```python
from build123d import *

# Parameters (mm, degrees)
SKETCH2_W           = 24
SKETCH2_H           = 75
BOSS_EXTRUDE1_DEPTH = 8
FILLET1_R           = 12
SKETCH3_W           = 24.000000014
SKETCH3_H           = 30
BOSS_EXTRUDE2_DEPTH = 50
SKETCH4_W           = 42
SKETCH4_H           = 27.227537437
CUT_EXTRUDE1_DEPTH  = 24
FILLET2_R           = 7
CUT_EXTRUDE3_DEPTH  = 14
SKETCH6_R           = 3
BOSS_EXTRUDE3_DEPTH = 5
FILLET3_R           = 3
SKETCH7_R           = 2
CUT_EXTRUDE4_DEPTH  = 102.473144681
SKETCH8_R           = 3
CUT_EXTRUDE5_DEPTH  = 4
SKETCH9_R           = 2
CUT_EXTRUDE6_DEPTH  = 10
FILLET4_R           = 7.5


# Some blends are built 0.0001 mm under size
with BuildPart() as part:
    # Sketch2 → Boss-Extrude1 (new body)
    with BuildSketch(Plane(origin=(0, -0.00023232, -27.997849314), x_dir=(1.0, -2.2299085471311813e-10, 0), z_dir=(-1.0101845712424022e-15, -8.29778911543011e-06, -0.9999999999655734))):
        with Locations((57.195219243, 10.372982491)):
            Rectangle(SKETCH2_W, SKETCH2_H)
    extrude(amount=BOSS_EXTRUDE1_DEPTH)

    # Fillet1
    # the kernel refuses this fillet: 12 mm, written as the material it takes off along each edge
    with BuildSketch(Plane(origin=(45.195219249, 27.127034112, 2.001925591), x_dir=(1.0, -2.229911070638136e-10, 0), z_dir=(-1.0101845712424022e-15, -8.29778911543011e-06, -0.9999999999655734))) as fillet1_piece_1:
        with BuildLine():
            CenterArc((FILLET1_R, FILLET1_R), FILLET1_R, 180, 90)
            Line((0, FILLET1_R), (0, 0))
            Line((0, 0), (FILLET1_R, 0))
        make_face()
    extrude(amount=68, mode=Mode.SUBTRACT)
    with BuildSketch(Plane(origin=(69.195219249, 27.127034106, 2.001925591), x_dir=(-1.0, 2.229905149399539e-10, 0), z_dir=(-1.0101845712424022e-15, -8.29778911543011e-06, -0.9999999999655734))) as fillet1_piece_2:
        with BuildLine():
            CenterArc((FILLET1_R, -FILLET1_R), FILLET1_R, 90, 90)
            Line((0, -FILLET1_R), (0, 0))
            Line((0, 0), (FILLET1_R, 0))
        make_face()
    extrude(amount=68, mode=Mode.SUBTRACT)

    # Sketch3 → Boss-Extrude2 (add)
    with BuildSketch(Plane(origin=(0, -0.00023232, -27.997849314), x_dir=(1, 0, 0), z_dir=(0, 8.297789115425485e-06, 0.9999999999655734))):
        with Locations((57.19521924, -32.872982501)):
            Rectangle(SKETCH3_W, SKETCH3_H)
    extrude(amount=BOSS_EXTRUDE2_DEPTH)

    # Sketch4 → Cut-Extrude1 (cut)
    with BuildSketch(Plane(origin=(69.195219243, -1.5e-08, 0), x_dir=(0, 0, -1), z_dir=(1.0, -2.2299088501705893e-10, 0))):
        with Locations((6.99770101, -40.486956155)):
            Rectangle(SKETCH4_W, SKETCH4_H)
    extrude(amount=-CUT_EXTRUDE1_DEPTH, mode=Mode.SUBTRACT)

    # Fillet2
    fillet2_edges = [part.edges().sort_by_distance(p)[0] for p in [
        (57.19521924, -17.87321482, -27.997701008),
        (57.19521924, -17.872799931, 22.002298991),
    ]]
    fillet(fillet2_edges, radius=FILLET2_R)

    # Sketch5 → Cut-Extrude3 (cut)
    with BuildSketch(Plane(origin=(69.195219243, -1.5e-08, 0), x_dir=(0, 0, -1), z_dir=(1.0, -2.2299088501705893e-10, 0))):
        Polygon((-22.002373674, -26.873187436), (-22.002547924, -47.872799915), (35.997452074, -47.873281192), (35.997626328, -26.873187436), align=None)
    extrude(amount=-CUT_EXTRUDE3_DEPTH, mode=Mode.SUBTRACT)

    # Sketch6 → Boss-Extrude3 (add)
    with BuildSketch(Plane(origin=(69.195219243, -1.5e-08, 0), x_dir=(0, 0, -1), z_dir=(1.0, -2.2299088501705893e-10, 0))):
        with BuildLine():
            Line((21.034070668, -17.873062539), (9.647551643, -17.873062539))
            Line((9.647551643, -17.873062539), (9.647551643, -47.873062539))
            Line((9.647551643, -47.873062539), (24.647551644, -47.873187436))
            Line((24.647551644, -47.873187436), (24.647551644, -16.846348023))
            ThreePointArc((24.647551644, -16.846348023), (22.910970159, -17.606627105), (21.034070668, -17.873062539))
        make_face()
        with Locations(Location((17.147551644, -37.873187436, 0), (0, 0, 270))):
            Circle(SKETCH6_R, mode=Mode.SUBTRACT)
    extrude(amount=BOSS_EXTRUDE3_DEPTH)

    # Fillet3
    fillet3_edges = [part.edges().sort_by_distance(p)[0] for p in [
        (45.195219233, -47.872833122, 18.002423457),
        (45.195219233, -47.873248012, -31.997576542),
    ]]
    fillet(fillet3_edges, radius=FILLET3_R)

    # Sketch7 → Cut-Extrude4 (cut, through all)
    with BuildSketch(Plane(origin=(0, -0.00023232, -27.997849314), x_dir=(1, 0, 0), z_dir=(0, 8.297789115402354e-06, 0.9999999999655734))):
        with Locations(Location((57.195219247, 15.127017497, 0), (0, 0, 270))):
            Circle(SKETCH7_R)
    extrude(amount=-CUT_EXTRUDE4_DEPTH, mode=Mode.SUBTRACT)

    # Sketch8 → Cut-Extrude5 (cut)
    with BuildSketch(Plane(origin=(0, -0.000298703, -35.997849314), x_dir=(-1, 0, 0), z_dir=(0, -8.297789115402354e-06, -0.9999999999655734))):
        with Locations(Location((-57.195219247, 15.127017497, 0), (0, 0, 90))):
            Circle(SKETCH8_R)
    extrude(amount=-CUT_EXTRUDE5_DEPTH, mode=Mode.SUBTRACT)

    # Sketch9 → Cut-Extrude6 (cut)
    with BuildSketch(Plane(origin=(55.195219243, -1.2e-08, 0), x_dir=(0, 0, -1), z_dir=(1.0, -2.2299126401379802e-10, 0))):
        with Locations(Location((31.29770101, -42.773187436, 0), (0, 0, 90))):
            Circle(SKETCH9_R)
        with Locations(Location((31.29770101, -32.973187436, 0), (0, 0, 90))):
            Circle(SKETCH9_R)
        with Locations(Location((-17.30229899, -42.773187436, 0), (0, 0, 90))):
            Circle(SKETCH9_R)
        with Locations(Location((-17.30229899, -32.973187436, 0), (0, 0, 90))):
            Circle(SKETCH9_R)
    extrude(amount=-CUT_EXTRUDE6_DEPTH, mode=Mode.SUBTRACT)

    # Fillet4
    fillet4_edges = [part.edges().sort_by_distance(p)[0] for p in [
        (71.695219233, -47.873187452, -24.647551644),
        (71.695219233, -47.873062555, -9.647551643),
    ]]
    fillet(fillet4_edges, radius=FILLET4_R - 0.0001)  # a hair under: the kernel refuses the full size


solid = part.part
```
Could you check a few things on this model? Use its own coordinates, in mm. A direction names the side the tool comes from. Coordinates: 2 decimals unless noted, no trailing zeros. Write each loop counter-clockwise with the first axis right and the second up, starting at its lowest first coordinate (ties: lowest second). Pieces come first, ordered by that corner, then holes. Notation, with made-up numbers: (16.25, 49) -> (64.25, 49) arc R20 cw to (64.25, 69) -> close; hole circle Ø3 at (81, 18). An arc over 180 degrees is marked (long way). Return JSON: item names as keys, results as strings.
(1) Which directions (+Z, -Z, +X, -X, +Y, -Y) give clear straight access to the entire face, cutting with the end or side of a thin tool? Please do faces 1 (the flat face through (72, -17.873, -15)), 2 (the flat face through (55.195, -37, 18)), 3 (the flat face through (72, -29, -24.648)).
Numbers:
{"face 1": "+Z, +X, -X, +Y", "face 2": "+Z, -Z, +X, -Y", "face 3": "-Z, +X, +Y, -Y"}
(2) I'm going to push flat-ended pins straight in: pin 1 (3 mm diameter, centred on x = 51, z = -9.5, fed in from +Y); pin 2 (2.5 mm diameter, centred on y = -23, z = 10.5, fed in from +X); pin 3 (12 mm diameter, centred on x = 52.5, y = 9, fed in from +Z); pin 4 (5.5 mm diameter, centred on y = -37.87, z = -17.15, fed in from -X). Where does each tip first touch, or does it pass through?
Numbers:
{"pin 1": "stops at y = -17.87", "pin 2": "stops at x = 69.2", "pin 3": "stops at z = -28", "pin 4": "passes through"}
(3) Imagine slicing it at A-A, the plane x = 52. Please give me the cut outline in (y, z).
Numbers:
{"outline": "(-47.87, -36) -> (25.94, -36) -> (25.94, -28) -> (-10.87, -28) arc R7 cw to (-17.87, -21) -> (-17.87, 15) arc R7 ccw to (-24.87, 22) -> (-47.87, 22) -> (-47.87, 14) -> (-26.87, 14) -> (-26.87, -28) -> (-47.87, -28) -> close; hole circle Ø4 at (-42.77, -31.3); hole circle Ø4 at (-42.77, 17.3); hole circle Ø4 at (-32.97, -31.3); hole circle Ø4 at (-32.97, 17.3)"}
(4) We'd pull the mould along Y, two halves only. Please class faces 4 (the cylindrical face through (50.27, -44.77, -31.21)), 5 (the flat face through (50, -38, -27.998)), 6 (the cylindrical face through (56.931, 27.124, -31.942)): +Y half, -Y half, draft (parallel to the pull), parting line (faces both ways), or undercut.
Numbers:
{"face 4": "undercut", "face 5": "draft", "face 6": "+Y half"}
(5) Imagine slicing it at C-C, the plane x = 63.25. Please give me the cut outline in (y, z), then the cut area to 3 significant figures.
Numbers:
{"outline": "(-26.87, -36) -> (25.49, -36) -> (25.49, -28) -> (-10.87, -28) arc R7 cw to (-17.87, -21) -> (-17.87, 15) arc R7 ccw to (-24.87, 22) -> (-26.87, 22) -> close", "area": "869 mm2"}
(6) I need wall thicknesses on L1, parallel to Y at x = 49.5, z = -32.5; L2, parallel to X at y = -34, z = -11; L3, parallel to Y at x = 49.75, z = -30. Which ranges of each line are inside material? Lowest first, please.
Numbers:
{"L1": "y = -47.87 to -44.37, -41.17 to -34.57, -31.37 to 24.33", "L2": "x = 69.2 to 74.2", "L3": "y = -47.87 to -44.3, -41.25 to -34.5, -31.45 to 24.54"}
(7) Imagine slicing it at D-D, the plane y = -21. Please give me the cut outline in (x, z).
Numbers:
{"outline": "(45.2, -36) -> (69.2, -36) -> (69.2, -24.65) -> (74.2, -24.65) -> (74.2, -9.65) -> (69.2, -9.65) -> (69.2, 20.83) -> (45.2, 20.83) -> close"}
